from build123d import *

# Parameters (mm, degrees)
F1_DEPTH = 10
F2_R     = 1.5
F3_DEPTH = 25
F4_R     = 3


with BuildPart() as f1:
    # F0 (on Top) → F1 (new body)
    with BuildSketch(Plane.XY):
        with BuildLine():
            Line((-26.545639, 48.637496), (-44.382463, 48.637496))
            ThreePointArc((-44.382463, 48.637496), (-47.917997, 47.17303), (-49.382463, 43.637496))
            Line((-49.382463, 43.637496), (-49.382463, 40.887496))
            Line((-49.382463, 40.887496), (-57.040692, 40.887496))
            Line((-57.040692, 40.887496), (-57.040692, 36.387496))
            Line((-57.040692, 36.387496), (-49.382463, 36.387496))
            Line((-49.382463, 36.387496), (-49.382463, 33.637496))
            ThreePointArc((-49.382463, 33.637496), (-47.917997, 30.101962), (-44.382463, 28.637496))
            Line((-44.382463, 28.637496), (-26.545639, 28.637496))
            Line((-26.545639, 28.637496), (-26.545639, 31.637496))
            Line((-26.545639, 31.637496), (-36.545639, 31.637496))
            Line((-36.545639, 31.637496), (-36.545639, 45.637496))
            Line((-36.545639, 45.637496), (-26.545639, 45.637496))
            Line((-26.545639, 45.637496), (-26.545639, 48.637496))
        make_face()
    extrude(amount=F1_DEPTH)

    # F2 (on face) → F3 (cut)
    with BuildSketch(Plane(origin=(0, 48.637496, 0), x_dir=(-1, 0, 0), z_dir=(0, 1, 0))):
        with Locations((54.540692, 5)):
            Circle(F2_R)
        with Locations((29.545639, 5)):
            Circle(F2_R)
    extrude(amount=-F3_DEPTH, mode=Mode.SUBTRACT)

    # F4
    f4_edges = [f1.edges().sort_by_distance(p)[0] for p in [
        (-57.040692, 38.637496, 10),
        (-57.040692, 38.637496, 0),
        (-26.545639, 47.137496, 10),
        (-26.545639, 30.137496, 10),
        (-26.545639, 47.137496, 0),
        (-26.545639, 30.137496, 0),
    ]]
    fillet(f4_edges, radius=F4_R)


solid = f1.part
The listing builds one solid part. Answer for the finished solid, in the listing's coordinates (mm). A direction names the side the tool comes from. Give positions to 0.01 mm unless a question says otherwise; leave off trailing zeros. Write each loop counter-clockwise with the first axis right and the second up, starting at its lowest first coordinate (ties: lowest second). Pieces come first, ordered by that corner, then holes.
Item 1: Section C-C, the plane y = 40.5 is taken. Write down the section's boundary in (x, z), plus the area to 3 significant figures.
Item 2: Which of the six approach directions +Z, -Z, +X, -X, +Y, -Y give full straight-line access (tool end or side, diameter ignored) to faces 4 (the flat face through (-42, 39, 0)), 5 (the flat face through (-49.382, 42, 5)), 6 (the flat face through (-52, 36.387, 5))?
Item 3: Section B-B, the plane z = 5 is taken. Write down the section's boundary in (x, y), plus the area to 3 significant figures.
Item 4: Section A-A, the plane x = -36 is taken. Write down the section's boundary in (y, z), plus the area to 3 significant figures.
Item 5: Flat-ended cylindrical pins translate along their axes: P1, Ø2, axis at y = 42, z = 5, coming from the -X side; P2, Ø4, axis at x = -53, z = 4, coming from the +Y side; P3, Ø2.5, axis at x = -54.54, z = 5, coming from the +Y side; P4, Ø5, axis at y = 39.5, z = 3, coming from the +X side. Find the tip coordinate at first contact, or state that the pin passes through.
Item 6: Section D-D, the plane x = -30.5 is taken. Write down the section's boundary in (y, z).
Item 7: Find the intervals of material crossed by line 1 along Y through (x, z) = (-34.5, 4.25); line 2 along Y through (x, z) = (-56, 7.75); line 3 along X through (y, z) = (33.75, 1.25), in increasing order.
Item 8: Determine the mould class of faces 1 (the flat face through (-36, 28.637, 5)), 2 (the cylindrical face through (-28.047, 47.158, 5.066)), 3 (the flat face through (-36.546, 39, 5)) for opening direction X: released by +X, released by -X, zero draft, split by the parting line, or undercut.
Completed:
1. outline: (-57.04, 3) arc R3 ccw to (-54.04, 0) - (-36.55, 0) - (-36.55, 10) - (-54.04, 10) arc R3 ccw to (-57.04, 7) - close; hole circle Ø3 at (-54.54, 5)
1. area: 194 mm2
2. face 4: -Z, +X, -X, +Y, -Y
2. face 5: +Z, -Z, -X, +Y
2. face 6: +Z, -Z, -X, -Y
3. outline: (-57.04, 36.39) - (-56.04, 36.39) - (-56.04, 40.89) - (-57.04, 40.89) - close; (-53.04, 36.39) - (-49.38, 36.39) - (-49.38, 33.64) arc R5 ccw to (-44.38, 28.64) - (-31.05, 28.64) - (-31.05, 31.64) - (-36.55, 31.64) - (-36.55, 45.64) - (-31.05, 45.64) - (-31.05, 48.64) - (-44.38, 48.64) arc R5 ccw to (-49.38, 43.64) - (-49.38, 40.89) - (-53.04, 40.89) - close; (-28.05, 28.64) - (-26.55, 28.64) - (-26.55, 31.64) - (-28.05, 31.64) - close; (-28.05, 45.64) - (-26.55, 45.64) - (-26.55, 48.64) - (-28.05, 48.64) - close
3. area: 309 mm2
4. outline: (28.64, 0) - (31.64, 0) - (31.64, 10) - (28.64, 10) - close; (45.64, 0) - (48.64, 0) - (48.64, 10) - (45.64, 10) - close
4. area: 60.0 mm2
5. P1: stops at x = -49.38
5. P2: stops at y = 40.89
5. P3: passes through
5. P4: stops at x = -36.55
6. outline: (28.64, 0) - (31.64, 0) - (31.64, 3.84) - (28.64, 3.84) - close; (28.64, 6.16) - (31.64, 6.16) - (31.64, 10) - (28.64, 10) - close; (45.64, 0) - (48.64, 0) - (48.64, 3.84) - (45.64, 3.84) - close; (45.64, 6.16) - (48.64, 6.16) - (48.64, 10) - (45.64, 10) - close
7. line 1: y = 28.64 to 31.64, 45.64 to 48.64
7. line 2: y = 36.39 to 40.89
7. line 3: x = -49.38 to -36.55
8. face 1: zero draft
8. face 2: undercut
8. face 3: released by +X
